For this review, use the dimensioned drawing (mm, ordinates from the lowest corner) and the shaded views. Round coordinates to 2 decimals unless told otherwise and drop trailing zeros. Write each loop counter-clockwise with the first axis right and the second up, starting at its lowest first coordinate (ties: lowest second). Pieces come first, ordered by that corner, then holes.
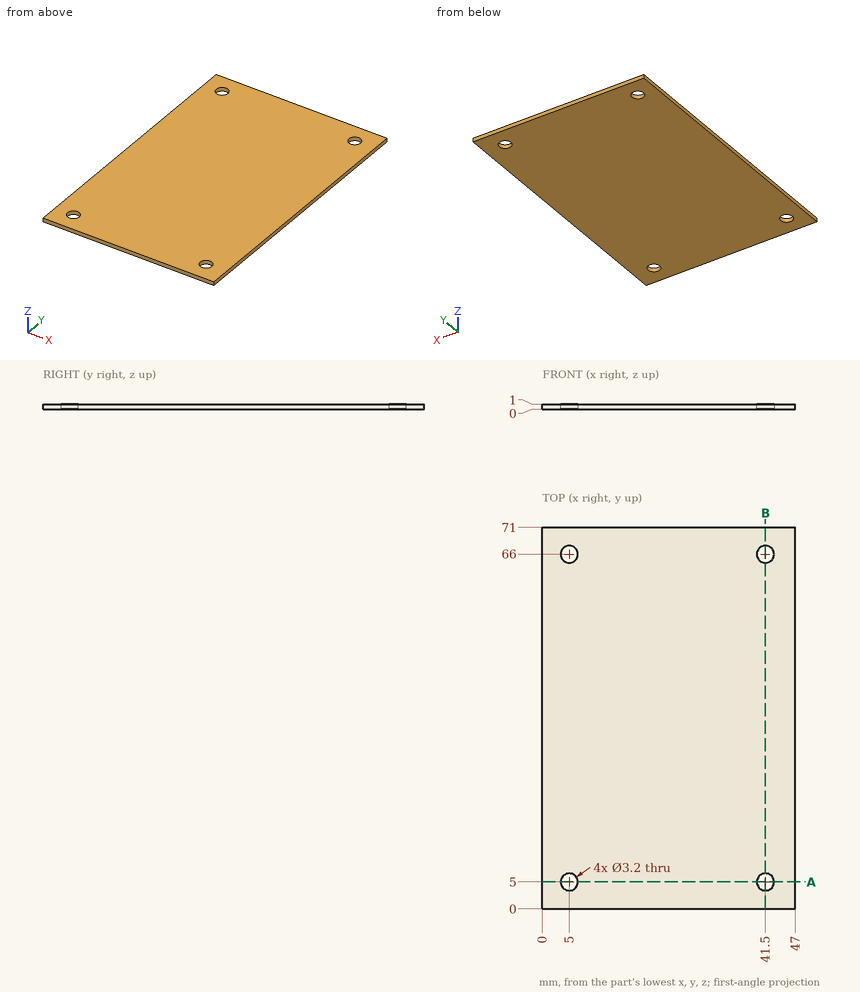
(1) We need section A-A, the plane y = 5. Give the boundary of the cut face in (x, z).
Geometry check:
outline: (0, 0) - (3.4, 0) - (3.4, 1) - (0, 1) - close; (6.6, 0) - (39.9, 0) - (39.9, 1) - (6.6, 1) - close; (43.1, 0) - (47, 0) - (47, 1) - (43.1, 1) - close
(2) For pin 1 Ø3.5 at (x, y) = (41.5, 66) entering from -Z, flat-tipped, find the tip position at first contact; note if it passes through.
Geometry check:
pin 1: stops at z = 0
(3) We need section B-B, the plane x = 41.5. Give the boundary of the cut face in (y, z), and give its area (3 significant figures).
Geometry check:
outline: (0, 0) - (3.4, 0) - (3.4, 1) - (0, 1) - close; (6.6, 0) - (64.4, 0) - (64.4, 1) - (6.6, 1) - close; (67.6, 0) - (71, 0) - (71, 1) - (67.6, 1) - close
area: 64.6 mm2
(4) For line 1 along Y through (x, z) = (5, 0.65), list the stretches that pass through material, from the lowest coordinate up.
Geometry check:
line 1: y = 0 to 3.4, 6.6 to 64.4, 67.6 to 71
